Autodesk Inventor part; units mm, degrees
ref_plane "YZ Plane" through (0, 0, 0) normal (1, 0, 0) x (0, 1, 0)
ref_plane "XZ Plane" through (0, 0, 0) normal (0, 1, 0) x (-1, 0, 0)
ref_plane "XY Plane" through (0, 0, 0) normal (0, 0, 1) x (1, 0, 0)
sketch "Sketch1" plane through (0, 0, 0) normal (0, 1, 0) x (-1, 0, 0)
  circle A0 centre (0, 0) radius 74.5 construction
  circle A1 centre (0, 30) radius 44.5 construction
  circle A2 centre (0, 30) radius 4.3
  circle A3 centre (0, 30) radius 10 construction
  arc A4 (9.8601, 31.6667) -> (-9.8601, 31.6667) centre (0, 30) ccw construction
  line L0 (0, -104.3) -> (0, 104.3) construction
  arc A5 (9.8601, 31.6667) -> (-9.8601, 31.6667) centre (0, 30) ccw
  line L1 (9.8601, 31.6667) -> (26.4003, -5.8228)
  arc A6 (-26.4003, -5.8228) -> (26.4003, -5.8228) centre (0, 30) ccw
  line L2 (-9.8601, 31.6667) -> (-26.4003, -5.8228)
  dimension "d5" = 20
  dimension "d0" = 149
  dimension "d3" = 30
  dimension "d4" = 8.6
extrude "Extrusion1" add sketch "Sketch1" along normal blind 1
sketch "Sketch2" plane through (0, 1, 0) normal (0, 1, 0) x (1, 0, 0)
  circle A0 centre (0, -30) radius 4.3 construction
  circle A1 centre (0, -30) radius 10.2
  point P0 (0, 0)
  dimension "d8" = 20.4
extrude "Extrusion2" cut sketch "Sketch2" against normal blind 0.5
sketch "Sketch3" plane through (0, 1, 0) normal (0, 1, 0) x (1, 0, 0)
  circle A0 centre (0, -30) radius 4.3 construction
  line L0 (9.8601, -31.6667) -> (26.4003, 5.8228) construction
  circle A1 centre (0, -30) radius 4.3 construction
  arc A2 (25.9919, 4.2553) -> (-25.7794, 4.4155) centre (0, -30) ccw
  arc A3 (14.5062, -21.136) -> (-14.5062, -21.136) centre (0, -30) ccw
  line L1 (14.5062, -21.136) -> (25.9919, 4.2553)
  line L2 (-26.4003, 5.8228) -> (-9.8601, -31.6667)
  line L3 (-14.5062, -21.136) -> (-25.7794, 4.4155)
  point P0 (0, 0)
  point P1 (-25.7794, 4.4155)
  dimension "d12" = 43
  dimension "d13" = 17
extrude "Extrusion3" cut sketch "Sketch3" against normal blind 0.4
properties part number "shutter"
The listing builds one solid part. Answer for the finished solid, in the listing's coordinates (mm). A direction names the side the tool comes from. Give positions to 0.01 mm unless a question says otherwise; leave off trailing zeros. Write each loop counter-clockwise with the first axis right and the second up, starting at its lowest first coordinate (ties: lowest second). Pieces come first, ordered by that corner, then holes.
1) Given P1, Ø1.5, axis at x = -6.5, z = -6, coming from the +Y side; P2, Ø16, axis at x = -1.5, z = 30.5, coming from the +Y side, each flat-ended and moving along its own axis, determine where each tip first touches the part or whether it passes through.
2) Section A-A (x = 0) is taken. Write down the section's boundary in (y, z).
3) Section D-D (z = -9) is taken. Write down the section's boundary in (x, y).
4) For a pull along Z with two mould halves and no side action, classify faces 1 (the face through (0, 1, 18)), 2 (the face through (0.196, 0.246, 39.998)), 3 (the face through (0.2, 0.8, 13)) as pulls with the +Z half, pulls with the -Z half, needs draft (parallel to the pull), parting line crosses it, or undercut.
5) A tool of negligible diameter and unlimited length cuts with its end or side. For faces 4 (the face through (0, 0.6, 0)), 5 (the face through (4, 0.5, 32)), 6 (the face through (-16.2, 0.4, 17.3)), from which of +Z, -Z, +X, -X, +Y, -Y can it reach the whole face along a straight path? Write none if from no direction.
6) Section B-B (y = 0.25) is taken. Write down the section's boundary in (x, z), and give its area (3 significant figures).
7) Section C-C (z = 30) is taken. Write down the section's boundary in (x, y).
8) Find the intervals of material crossed by L1, parallel to Z at x = 0, y = 0.3; L2, parallel to Y at x = 3, z = 21.5; L3, parallel to X at y = 0.6, z = 22.5, in increasing order.
Response:
1. P1: stops at y = 0.6
1. P2: stops at y = 0.5
2. outline: (0, -14.5) - (1, -14.5) - (1, -13) - (0.6, -13) - (0.6, 13) - (1, 13) - (1, 19.8) - (0.5, 19.8) - (0.5, 25.7) - (0, 25.7) - close; (0, 34.3) - (0.5, 34.3) - (0.5, 40) - (0, 40) - close
3. outline: (-21.43, 0) - (21.43, 0) - (21.43, 1) - (18.11, 1) - (18.11, 0.6) - (-18.11, 0.6) - (-18.11, 1) - (-21.43, 1) - close
4. face 1: needs draft
4. face 2: pulls with the +Z half
4. face 3: undercut
5. face 4: +Y
5. face 5: +Z, +Y
5. face 6: +Z, -X, +Y, -Y
6. outline: (-26.4, -5.82) arc R44.5 ccw to (26.4, -5.82) - (9.86, 31.67) arc R10 ccw to (-9.86, 31.67) - close; hole circle Ø8.6 at (0, 30)
6. area: 1,740 mm2
7. outline: (-10.6, 0) - (-4.3, 0) - (-4.3, 0.5) - (-10.2, 0.5) - (-10.2, 1) - (-10.6, 1) - close; (4.3, 0) - (10.6, 0) - (10.6, 1) - (10.2, 1) - (10.2, 0.5) - (4.3, 0.5) - close
8. L1: z = -14.5 to 25.7, 34.3 to 40
8. L2: y = 0 to 0.5
8. L3: x = -13.9 to -6.91, 6.91 to 13.9
